```python
from build123d import *

# Parameters (mm, degrees)
F0_W     = 105.55536
F0_H     = 58.80253
F1_DEPTH = 76.2
F2_W     = 92.85536
F2_H     = 46.10253
F3_DEPTH = 76.2
F4_W     = 54.75536
F4_H     = 6.35
F5_DEPTH = 25.4
F6_R     = 12.7
F7_DEPTH = 25.4
F8_R     = 12.7
F9_DEPTH = 25.4


with BuildPart() as f1:
    # F0 (on Top) → F1 (new body)
    with BuildSketch(Plane.XY):
        with Locations((2.530435, -10.00125)):
            Rectangle(F0_W, F0_H)
    extrude(amount=F1_DEPTH)

    # F2 (on face) → F3 (cut, through all)
    with BuildSketch(Plane.XY.offset(76.2)):
        with Locations((2.530435, -10.00125)):
            Rectangle(F2_W, F2_H)
    extrude(amount=-F3_DEPTH, mode=Mode.SUBTRACT)

    # F4 (on face) → F5 (cut)
    with BuildSketch(Plane.XY.offset(76.2)):
        with Locations((2.530435, -36.227515)):
            Rectangle(F4_W, F4_H)
        with Locations((2.530435, 16.225015)):
            Rectangle(F4_W, F4_H)
    extrude(amount=-F5_DEPTH, mode=Mode.SUBTRACT)

    # F6 (on face) → F7 (cut)
    with BuildSketch(Plane.YZ.offset(55.308115)):
        with Locations((-11.462515, 38.1)):
            Circle(F6_R)
    extrude(amount=-F7_DEPTH, mode=Mode.SUBTRACT)

    # F8 (on face) → F9 (cut)
    with BuildSketch(Plane(origin=(-50.247245, 0, 0), x_dir=(0, -1, 0), z_dir=(-1, 0, 0))):
        with Locations((10.192515, 38.1)):
            Circle(F8_R)
    extrude(amount=-F9_DEPTH, mode=Mode.SUBTRACT)


solid = f1.part
```
Here's how the part is built. I have some questions about the finished solid (model axes, mm). A direction names the side the tool comes from. Round coordinates to 2 decimals unless told otherwise and drop trailing zeros. Loops run counter-clockwise (first coordinate to the right, second up) from the corner with the lowest first, then second, coordinate; pieces in that order, holes last. Notation, with made-up numbers: (20, -15) -> (62, -15) arc R22 cw to (62, -8) -> close; hole circle Ø1 at (67.25, 7). An arc over 180 degrees is marked (long way). Answer as CSV lines item,"result". Start each with the question number.
1. For faces 5 (the face through (52.18, -4.64, 48.81)), 6 (the face through (29.908, 16, 64)), 7 (the face through (2, 13.05, 30)), which set-ups out of +Z, -Z, +X, -X, +Y, -Y let a thin tool reach every point of the face, with its end or its side?
2. Imagine slicing it at C-C on x = 2.5. Write out the boundary of the cut face in (y, z), plus the area to 3 significant figures.
3. If we mould it in two halves opening along Y, with no side actions, what happens to faces 1 (the face through (48.958, 0, 47)), 2 (the face through (2, -39.403, 29)), 3 (the face through (2, 19.4, 29)), 4 (the face through (2, 14, 0))? For each: pulls with the +Y half, pulls with the -Y half, needs draft (parallel to the pull), parting line crosses it, or undercut.
4. Imagine slicing it at B-B on z = 38.1. Write out the boundary of the cut face in (x, y), plus the area to 3 significant figures.
5. Imagine slicing it at A-A on y = 8. Write out the boundary of the cut face in (x, z).
6. I'm going to push flat-ended pins straight in: P1, Ø3, axis at x = 0.5, y = 16, coming from the +Z side; P2, Ø20.5, axis at y = -10.19, z = 38.1, coming from the +X side. Where does each tip first touch, or does it pass through?
7. Imagine slicing it at D-D on y = -8. Write out the boundary of the cut face in (x, z), plus the area to 3 significant figures.
8. I need wall thicknesses on probe 1 along Y at (x, z) = (-36, 41); probe 2 along X at (y, z) = (9.5, 67.5); probe 3 along Y at (x, z) = (-48, 38). Which ranges of each line are inside material? Lowest first, please. Write a range as from..to.
Solution:
1,face 5,"+X"
1,face 6,"+Z, +Y, -Y"
1,face 7,"+Z, -Z"
2,outline,"(-39.4, 0) -> (-33.05, 0) -> (-33.05, 50.8) -> (-39.4, 50.8) -> close; (13.05, 0) -> (19.4, 0) -> (19.4, 50.8) -> (13.05, 50.8) -> close"
2,area,"645 mm²"
3,face 1,"undercut"
3,face 2,"pulls with the -Y half"
3,face 3,"pulls with the +Y half"
3,face 4,"needs draft"
4,outline,"(-50.25, -39.4) -> (55.31, -39.4) -> (55.31, -24.16) -> (48.96, -24.16) -> (48.96, -33.05) -> (-43.9, -33.05) -> (-43.9, -22.89) -> (-50.25, -22.89) -> close; (-50.25, 2.51) -> (-43.9, 2.51) -> (-43.9, 13.05) -> (48.96, 13.05) -> (48.96, 1.24) -> (55.31, 1.24) -> (55.31, 19.4) -> (-50.25, 19.4) -> close"
4,area,"1,600 mm²"
5,outline,"(-50.25, 0) -> (-43.9, 0) -> (-43.9, 76.2) -> (-50.25, 76.2) -> close; (48.96, 0) -> (55.31, 0) -> (55.31, 76.2) -> (48.96, 76.2) -> close"
6,P1,"z = 50.8"
6,P2,"through"
7,outline,"(-50.25, 0) -> (-43.9, 0) -> (-43.9, 25.59) -> (-50.25, 25.59) -> close; (-50.25, 50.61) -> (-43.9, 50.61) -> (-43.9, 76.2) -> (-50.25, 76.2) -> close; (48.96, 0) -> (55.31, 0) -> (55.31, 25.88) -> (48.96, 25.88) -> close; (48.96, 50.32) -> (55.31, 50.32) -> (55.31, 76.2) -> (48.96, 76.2) -> close"
7,area,"654 mm²"
8,probe 1,"-39.4..-33.05, 13.05..19.4"
8,probe 2,"-50.25..-43.9, 48.96..55.31"
8,probe 3,"-39.4..-22.89, 2.51..19.4"
